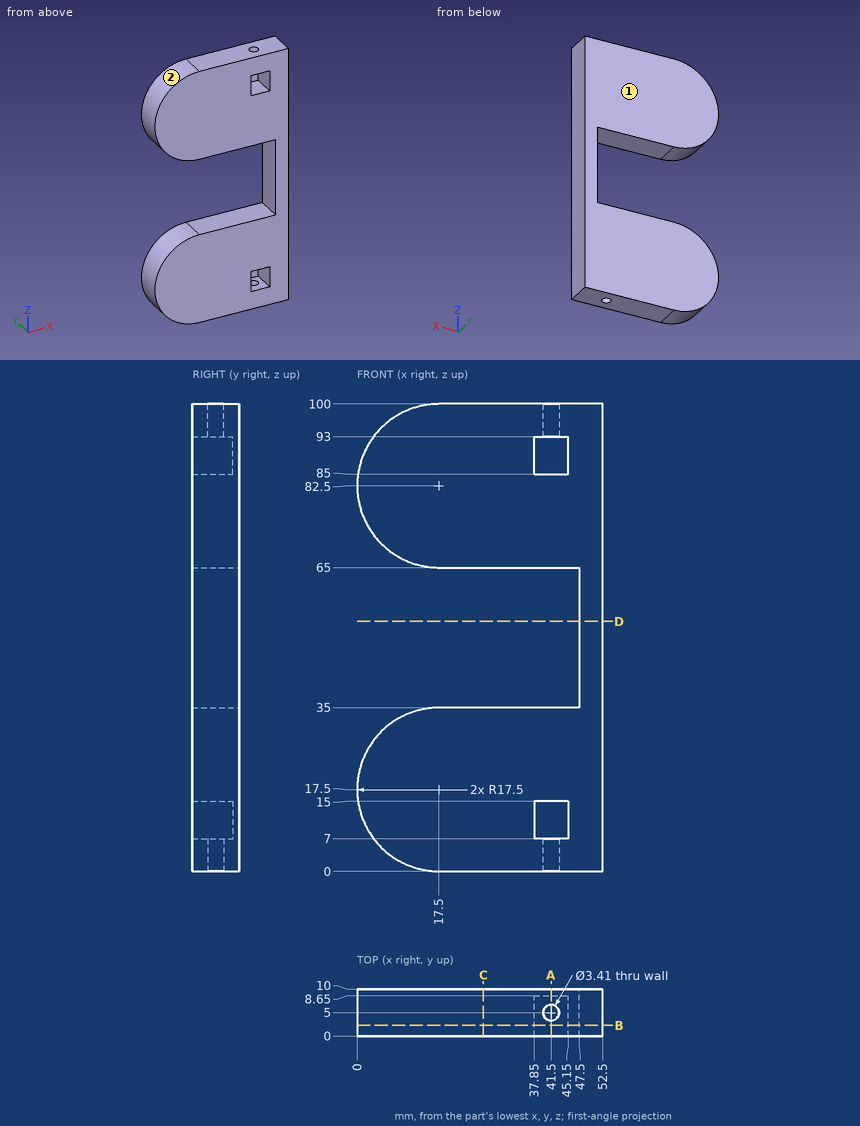
Job drawing, mm, ordinate dimensions from the low corner. One solid piece. Round coordinates to 2 decimals unless told otherwise and drop trailing zeros. Order: outer loops, then holes, each group sorted by start corner. A loop starts at its lowest first (then second) coordinate and runs counter-clockwise, first axis right, second up. Notation, with made-up numbers: M 24.25,55.25 L 46.25,55.25 A12 cw 46.25,63.25 Z; hole C 25,67 d7. An arc over 180 degrees is marked long. Write each question's results on one line, items separated by ' | '. Start each with the question number.
(1) Saw through at C-C, the plane x = 27. Give the cut face in (y, z).
(2) Drop flat-ended pins along their axis: pin 1 (2 mm diameter, centred on x = 6, y = 5, fed in from -Z); pin 2 (2.5 mm diameter, centred on x = 41.5, y = 5, fed in from +Z); pin 3 (1 mm diameter, centred on x = 13, y = 5, fed in from -Z); pin 4 (3 mm diameter, centred on x = 25, z = 37, fed in from +Y). Give the stop position or say it passes through.
(3) Probe probe 1 along Z at (x, y) = (45.5, 0.75); probe 2 along Z at (x, y) = (38, 3.5); probe 3 along X at (y, z) = (4.5, 43.5). List the from-to ranges inside material, lowest first. Write a range as from..to.
(4) Saw through at B-B, the plane y = 2.25. Give the cut face in (x, z).
(5) Two-plate mould, pull along Z, no slides. Class the marked faces 1 and 2: pulls with the +Z half, pulls with the -Z half, needs draft (parallel to the pull), parting line crosses it, or undercut.
(6) Saw through at D-D, the plane z = 53.5. Give the cut face in (x, y), then the cut area to 3 significant figures.
(7) Saw through at A-A, the plane x = 41.5. Give the cut face in (y, z) (3 decimals).
Established:
1) outline: M 0,0 L 10,0 L 10,35 L 0,35 Z; M 0,65 L 10,65 L 10,100 L 0,100 Z
2) pin 1: stops at z = 3.5 | pin 2: stops at z = 85 | pin 3: stops at z = 0.46 | pin 4: passes through
3) probe 1: z = 0..35, 65..100 | probe 2: z = 0..7, 15..35, 65..85, 93..100 | probe 3: x = 47.5..52.5
4) outline: M 17.5,0 L 52.5,0 L 52.5,100 L 17.5,100 A17.5 ccw 17.5,65 L 47.5,65 L 47.5,35 L 17.5,35 A17.5 ccw Z; hole M 37.85,7 L 45.15,7 L 45.15,15 L 37.85,15 Z; hole M 37.85,85 L 45.15,85 L 45.15,93 L 37.85,93 Z
5) face 1: needs draft | face 2: undercut
6) outline: M 47.5,0 L 52.5,0 L 52.5,10 L 47.5,10 Z | area: 50.0 mm^2
7) outline: M 0,0 L 3.295,0 L 3.295,7 L 0,7 Z; M 0,15 L 8.65,15 L 8.65,7 L 6.705,7 L 6.705,0 L 10,0 L 10,35 L 0,35 Z; M 0,65 L 10,65 L 10,100 L 6.705,100 L 6.705,93 L 8.65,93 L 8.65,85 L 0,85 Z; M 0,93 L 3.295,93 L 3.295,100 L 0,100 Z
